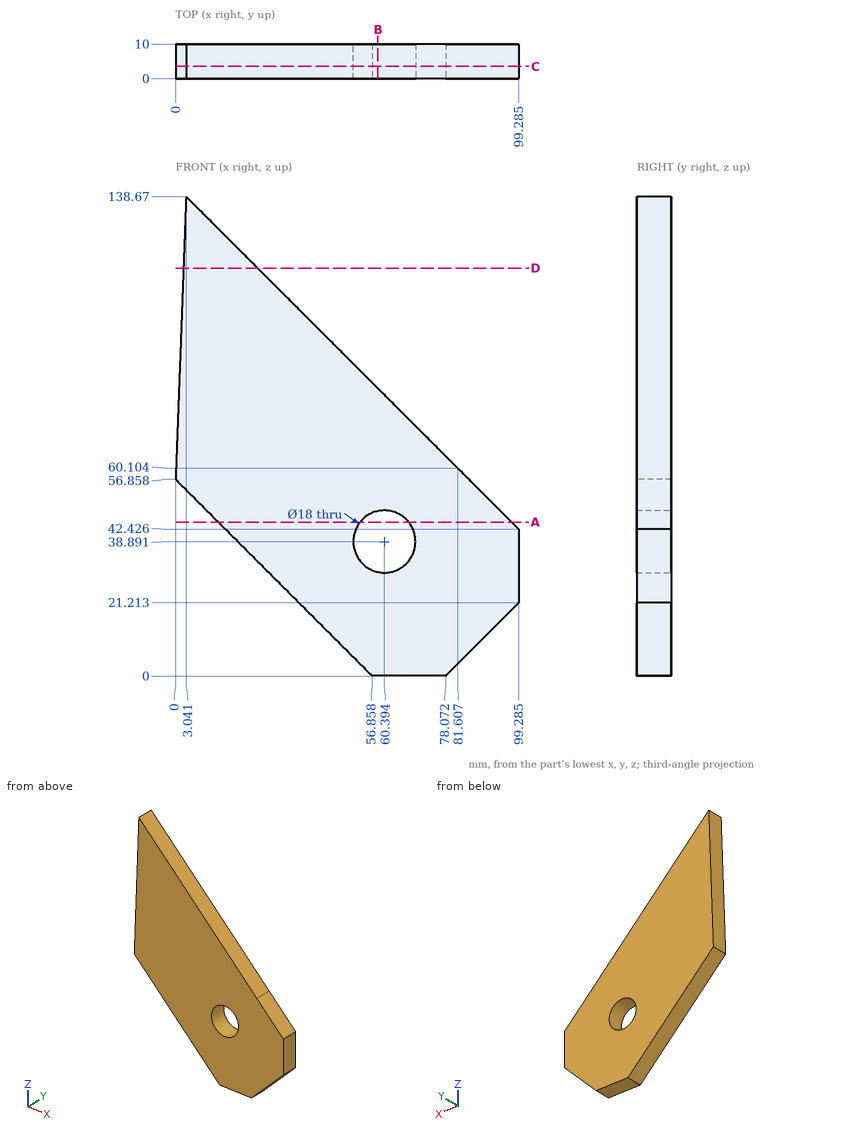
Geometry check sheet. Reference: drawing and pictorial views, mm from the part's lowest x, y, z. Round coordinates to 2 decimals unless told otherwise and drop trailing zeros. Loops run counter-clockwise (first coordinate to the right, second up) from the corner with the lowest first, then second, coordinate; pieces in that order, holes last. Notation, with made-up numbers: (-17.5, -37) - (-13.5, -37) arc R23 ccw to (-13.5, -17) - close; hole circle Ø10 at (-36.5, 72). An arc over 180 degrees is marked (long way). Write item = value, one per line. Start each with the question number.
Q1. Section check A-A (z = 44.5). Record the boundary of the cut face in (x, y) (1 decimal), plus the area to 3 significant figures.
Q2. Thickness scan on L1, parallel to Z at x = 68, y = 1.5 (1 decimal); L2, parallel to Z at x = 60, y = 8.5; L3, parallel to X at y = 5, z = 45 (1 decimal). Record the ranges inside material, lowest first.
Q3. Section check D-D (z = 118). Record the boundary of the cut face in (x, y), plus the area to 3 significant figures.
Q4. Depth check by flat-ended pin: P1, Ø3, axis at y = 8, z = 23, coming from the -X side; P2, Ø16, axis at x = 60.39, z = 38.89, coming from the +Y side; P3, Ø3, axis at x = 23, y = 7, coming from the +Z side; P4, Ø1, axis at x = 29, y = 9, coming from the -Z side. Enter the tip coordinate at first touch or a pass-through.
Q5. Section check B-B (x = 58.5). Record the boundary of the cut face in (y, z).
Q6. Section check C-C (y = 3.5). Record the boundary of the cut face in (x, z) (1 decimal).
Derived:
q1.outline = (12.4, 0) - (53.4, 0) - (53.4, 10) - (12.4, 10) - close; (67.4, 0) - (97.2, 0) - (97.2, 10) - (67.4, 10) - close
q1.area = 708 mm^2
q2.L1 = 0 to 34.1, 43.7 to 73.7
q2.L2 = 0 to 29.9, 47.88 to 81.71
q2.L3 = 11.9 to 53.8, 67 to 96.7
q3.outline = (2.27, 0) - (23.71, 0) - (23.71, 10) - (2.27, 10) - close
q3.area = 214 mm^2
q4.P1 = 32.36
q4.P2 = through
q4.P3 = 120.21
q4.P4 = 27.36
q5.outline = (0, 0) - (10, 0) - (10, 30.09) - (0, 30.09) - close; (0, 47.69) - (10, 47.69) - (10, 83.21) - (0, 83.21) - close
q6.outline = (0, 56.9) - (56.9, 0) - (78.1, 0) - (99.3, 21.2) - (99.3, 42.4) - (3, 138.7) - close; hole circle Ø18 at (60.4, 38.9)
